Verification items for the finished model (mm, model axes). A direction names the side the tool comes from. Give positions to 0.01 mm unless a question says otherwise; leave off trailing zeros. Use CSV: the item, a comma, the result in double quotes.
from build123d import *

# Parameters (mm, degrees)
F2_W     = 45
F2_H     = 10.7396448086
F3_DEPTH = 2
F0_W     = 45
F0_H     = 10.7396448086
F4_DEPTH = 1


with BuildPart() as f3:
    # F2 (on offset) → F3 (new body)
    with BuildSketch(Plane.XY.offset(-2)):
        with Locations((20.6953600791, -3.6390531603)):
            Rectangle(F2_W, F2_H)
    extrude(amount=F3_DEPTH)

    # F0 (on Top) → F4 (join)
    with BuildSketch(Plane.XY):
        with Locations((20.6953600791, -3.6390531603)):
            Rectangle(F0_W, F0_H)
        Polygon((3.1538346612, -0.7923350599), (3.1538346612, -7.1449705598), (2.3304884443, -7.1449705598), (2.3304884443, -0.7923350599), (0.0868312394, -0.7923350599), (0.0868312394, -0.060471756), (5.397491866, -0.060471756), (5.397491866, -0.7923350599), align=None, mode=Mode.SUBTRACT)
        with BuildLine():
            add(Edge.make_bspline(
                [(11.7563295973, -0.9179302455), (12.6137880868, -1.8870289), (12.6137880868, -3.5926425319)],
                knots=[0, 0, 0, 1, 1, 1], degree=2))
            add(Edge.make_bspline(
                [(12.6137880868, -3.5926425319), (12.6137880868, -5.2936044903), (11.7532284816, -6.2681300972)],
                knots=[0, 0, 0, 1, 1, 1], degree=2))
            add(Edge.make_bspline(
                [(11.7532284816, -6.2681300972), (10.8926688764, -7.2426557042), (9.3622682813, -7.2426557042)],
                knots=[0, 0, 0, 1, 1, 1], degree=2))
            add(Edge.make_bspline(
                [(9.3622682813, -7.2426557042), (7.7977554135, -7.2426557042), (6.9472744343, -6.2851862335)],
                knots=[0, 0, 0, 1, 1, 1], degree=2))
            add(Edge.make_bspline(
                [(6.9472744343, -6.2851862335), (6.0967934551, -5.3277167629), (6.0967934551, -3.5833391848)],
                knots=[0, 0, 0, 1, 1, 1], degree=2))
            add(Edge.make_bspline(
                [(6.0967934551, -3.5833391848), (6.0967934551, -1.8529166274), (6.9496002711, -0.9008741092)],
                knots=[0, 0, 0, 1, 1, 1], degree=2))
            add(Edge.make_bspline(
                [(6.9496002711, -0.9008741092), (7.802407087, 0.051168409), (9.3715716284, 0.051168409)],
                knots=[0, 0, 0, 1, 1, 1], degree=2))
            add(Edge.make_bspline(
                [(9.3715716284, 0.051168409), (10.8988711078, 0.051168409), (11.7563295973, -0.9179302455)],
                knots=[0, 0, 0, 1, 1, 1], degree=2))
        make_face(mode=Mode.SUBTRACT)
        with BuildLine():
            Line((22.2706623591, -0.060471756), (20.3758806698, -7.1449705598))
            Line((20.3758806698, -7.1449705598), (19.5618378, -7.1449705598))
            Line((19.5618378, -7.1449705598), (18.1322234649, -2.4018141053))
            add(Edge.make_bspline(
                [(18.1322234649, -2.4018141053), (18.029886647, -2.0855003045), (17.9042914614, -1.6063779297)],
                knots=[0, 0, 0, 1, 1, 1], degree=2))
            add(Edge.make_bspline(
                [(17.9042914614, -1.6063779297), (17.7786962758, -1.1272555549), (17.7740446022, -1.0295704105)],
                knots=[0, 0, 0, 1, 1, 1], degree=2))
            add(Edge.make_bspline(
                [(17.7740446022, -1.0295704105), (17.6670561108, -1.6699508014), (17.4344724337, -2.4297241465)],
                knots=[0, 0, 0, 1, 1, 1], degree=2))
            Line((17.4344724337, -2.4297241465), (16.0482737183, -7.1449705598))
            Line((16.0482737183, -7.1449705598), (15.2342308486, -7.1449705598))
            Line((15.2342308486, -7.1449705598), (13.3487525064, -0.060471756))
            Line((13.3487525064, -0.060471756), (14.2217165743, -0.060471756))
            Line((14.2217165743, -0.060471756), (15.34121934, -4.4361460008))
            add(Edge.make_bspline(
                [(15.34121934, -4.4361460008), (15.5738030171, -5.357177362), (15.6807915085, -6.1029956865)],
                knots=[0, 0, 0, 1, 1, 1], degree=2))
            add(Edge.make_bspline(
                [(15.6807915085, -6.1029956865), (15.8110383677, -5.2160765979), (16.0684309703, -4.3679214555)],
                knots=[0, 0, 0, 1, 1, 1], degree=2))
            Line((16.0684309703, -4.3679214555), (17.3367872893, -0.060471756))
            Line((17.3367872893, -0.060471756), (18.2097513573, -0.060471756))
            Line((18.2097513573, -0.060471756), (19.541680548, -4.4066854017))
            add(Edge.make_bspline(
                [(19.541680548, -4.4066854017), (19.7742642251, -5.1587059576), (19.9339716834, -6.1029956865)],
                knots=[0, 0, 0, 1, 1, 1], degree=2))
            add(Edge.make_bspline(
                [(19.9339716834, -6.1029956865), (20.0270051542, -5.4145480024), (20.282847199, -4.4268426537)],
                knots=[0, 0, 0, 1, 1, 1], degree=2))
            Line((20.282847199, -4.4268426537), (21.3976982911, -0.060471756))
            Line((21.3976982911, -0.060471756), (22.2706623591, -0.060471756))
        make_face(mode=Mode.SUBTRACT)
        Polygon((28.6853201729, -7.1449705598), (27.8325133569, -7.1449705598), (26.9502459419, -4.8920100079), (24.1111745237, -4.8920100079), (23.2397610136, -7.1449705598), (22.4055608918, -7.1449705598), (25.2058683638, -0.0310111569), (25.8989677215, -0.0310111569), align=None, mode=Mode.SUBTRACT)
        with BuildLine():
            Line((31.961648904, -4.1989106502), (30.4824167177, -4.1989106502))
            Line((30.4824167177, -4.1989106502), (30.4824167177, -7.1449705598))
            Line((30.4824167177, -7.1449705598), (29.6590705009, -7.1449705598))
            Line((29.6590705009, -7.1449705598), (29.6590705009, -0.060471756))
            Line((29.6590705009, -0.060471756), (31.6019194834, -0.060471756))
            add(Edge.make_bspline(
                [(31.6019194834, -0.060471756), (32.9059386329, -0.060471756), (33.5284876085, -0.5597513828)],
                knots=[0, 0, 0, 1, 1, 1], degree=2))
            add(Edge.make_bspline(
                [(33.5284876085, -0.5597513828), (34.1510365842, -1.0590310096), (34.1510365842, -2.0622419368)],
                knots=[0, 0, 0, 1, 1, 1], degree=2))
            add(Edge.make_bspline(
                [(34.1510365842, -2.0622419368), (34.1510365842, -3.4670473463), (32.7260739226, -3.9616752995)],
                knots=[0, 0, 0, 1, 1, 1], degree=2))
            Line((32.7260739226, -3.9616752995), (34.650316211, -7.1449705598))
            Line((34.650316211, -7.1449705598), (33.6765658829, -7.1449705598))
            Line((33.6765658829, -7.1449705598), (31.961648904, -4.1989106502))
        make_face(mode=Mode.SUBTRACT)
        Polygon((41.0990862974, -7.1449705598), (40.2462794814, -7.1449705598), (39.3640120664, -4.8920100079), (36.5249406482, -4.8920100079), (35.6535271381, -7.1449705598), (34.8193270163, -7.1449705598), (37.6196344883, -0.0310111569), (38.312733846, -0.0310111569), align=None, mode=Mode.SUBTRACT)
        with BuildLine():
            add(Edge.make_bspline(
                [(7.5814525938, -1.4296143351), (6.9682069652, -2.1738821017), (6.9682069652, -3.5926425319)],
                knots=[0, 0, 0, 1, 1, 1], degree=2))
            add(Edge.make_bspline(
                [(6.9682069652, -3.5926425319), (6.9682069652, -5.0315602141), (7.5814525938, -5.7758279808)],
                knots=[0, 0, 0, 1, 1, 1], degree=2))
            add(Edge.make_bspline(
                [(7.5814525938, -5.7758279808), (8.1946982224, -6.5200957474), (9.3622682813, -6.5200957474)],
                knots=[0, 0, 0, 1, 1, 1], degree=2))
            add(Edge.make_bspline(
                [(9.3622682813, -6.5200957474), (10.5391416873, -6.5200957474), (11.1399828531, -5.7789290964)],
                knots=[0, 0, 0, 1, 1, 1], degree=2))
            add(Edge.make_bspline(
                [(11.1399828531, -5.7789290964), (11.7408240189, -5.0377624455), (11.7408240189, -3.5926425319)],
                knots=[0, 0, 0, 1, 1, 1], degree=2))
            add(Edge.make_bspline(
                [(11.7408240189, -3.5926425319), (11.7408240189, -2.1630281968), (11.1423086898, -1.4241873826)],
                knots=[0, 0, 0, 1, 1, 1], degree=2))
            add(Edge.make_bspline(
                [(11.1423086898, -1.4241873826), (10.5437933608, -0.6853465685), (9.3715716284, -0.6853465685)],
                knots=[0, 0, 0, 1, 1, 1], degree=2))
            add(Edge.make_bspline(
                [(9.3715716284, -0.6853465685), (8.1946982224, -0.6853465685), (7.5814525938, -1.4296143351)],
                knots=[0, 0, 0, 1, 1, 1], degree=2))
        make_face()
        with BuildLine():
            Line((24.4026793989, -4.1508433569), (26.6944038971, -4.1508433569))
            Line((26.6944038971, -4.1508433569), (25.8695071224, -1.9552534453))
            add(Edge.make_bspline(
                [(25.8695071224, -1.9552534453), (25.7097996641, -1.5381533844), (25.5407888588, -0.933435824)],
                knots=[0, 0, 0, 1, 1, 1], degree=2))
            add(Edge.make_bspline(
                [(25.5407888588, -0.933435824), (25.4338003673, -1.3986031782), (25.2353289629, -1.9552534453)],
                knots=[0, 0, 0, 1, 1, 1], degree=2))
            Line((25.2353289629, -1.9552534453), (24.4026793989, -4.1508433569))
        make_face()
        with BuildLine():
            Line((30.4824167177, -0.7830317128), (30.4824167177, -3.4918562719))
            Line((30.4824167177, -3.4918562719), (31.6127733883, -3.4918562719))
            add(Edge.make_bspline(
                [(31.6127733883, -3.4918562719), (32.4841868985, -3.4918562719), (32.8912083333, -3.145306593)],
                knots=[0, 0, 0, 1, 1, 1], degree=2))
            add(Edge.make_bspline(
                [(32.8912083333, -3.145306593), (33.2982297682, -2.7987569142), (33.2982297682, -2.1056575565)],
                knots=[0, 0, 0, 1, 1, 1], degree=2))
            add(Edge.make_bspline(
                [(33.2982297682, -2.1056575565), (33.2982297682, -1.4032548517), (32.884230823, -1.0931432823)],
                knots=[0, 0, 0, 1, 1, 1], degree=2))
            add(Edge.make_bspline(
                [(32.884230823, -1.0931432823), (32.4702318778, -0.7830317128), (31.5538521901, -0.7830317128)],
                knots=[0, 0, 0, 1, 1, 1], degree=2))
            Line((31.5538521901, -0.7830317128), (30.4824167177, -0.7830317128))
        make_face()
        with BuildLine():
            Line((36.8164455235, -4.1508433569), (39.1081700216, -4.1508433569))
            Line((39.1081700216, -4.1508433569), (38.2832732469, -1.9552534453))
            add(Edge.make_bspline(
                [(38.2832732469, -1.9552534453), (38.1235657886, -1.5381533844), (37.9545549833, -0.933435824)],
                knots=[0, 0, 0, 1, 1, 1], degree=2))
            add(Edge.make_bspline(
                [(37.9545549833, -0.933435824), (37.8475664919, -1.3986031782), (37.6490950874, -1.9552534453)],
                knots=[0, 0, 0, 1, 1, 1], degree=2))
            Line((37.6490950874, -1.9552534453), (36.8164455235, -4.1508433569))
        make_face()
    extrude(amount=F4_DEPTH)


solid = f3.part
(1) Mould release check, pull along X, two halves, no side actions. Record for faces 3 (the flat face through (20, -4, 1)), 4 (the flat face through (43.195, -4, -1)), 5 (the flat face through (2.7, -7.145, 0.5)): released by +X, released by -X, zero draft, split by the parting line, or undercut.
Calculated:
face 3,"zero draft"
face 4,"released by +X"
face 5,"undercut"
(2) Section check A-A on z = 0.55. Count the separate pieces of the cut face and the enclosed holes in it, plus the area to 3 significant figures.
Calculated:
separate pieces,"5"
enclosed holes,"6"
area,"396 mm²"
(3) Scan lines: L1, parallel to Y at x = 1, z = 0.6; L2, parallel to Z at x = 15.5, y = -6.75. Record each from-to range of solid material in increasing order. Write a range as from..to.
Calculated:
L1,"y = -9.01..-0.79, -0.06..1.73"
L2,"z = -2..0"
(4) Tool access check on faces 1 (the flat face through (20, -9.009, -1)), 2 (the flat face through (13.8, -0.06, 0.5)). Record the directions out of +Z, -Z, +X, -X, +Y, -Y that give a thin tool (end or side, any length) a straight path to the whole face; none if there is none.
Calculated:
face 1,"+Z, -Z, +X, -X, -Y"
face 2,"+Z"
